Work out the finished part from the listing and answer in its coordinate system (mm). Round coordinates to 2 decimals unless told otherwise and drop trailing zeros. Order: outer loops, then holes, each group sorted by start corner. A loop starts at its lowest first (then second) coordinate and runs counter-clockwise, first axis right, second up. Notation, with made-up numbers: (73.25, -19.5) -> (120.25, -19.5) arc R21 cw to (120.25, -8.5) -> close; hole circle Ø10 at (14.25, 56). An arc over 180 degrees is marked (long way). Use one line per item in the form item = value.
```python
from build123d import *

# Parameters (mm, degrees)
F0_R     = 3.25
F0_R_2   = 0.335
F1_DEPTH = 57.25
F2_SIZE  = 2
F3_SIZE  = 1


with BuildPart() as f1:
    # F0 (on Top) → F1 (new body)
    with BuildSketch(Plane.XY):
        Circle(F0_R)
        Circle(F0_R_2, mode=Mode.SUBTRACT)
    extrude(amount=F1_DEPTH)

    # F2
    f2_edges = [f1.edges().sort_by_distance(p)[0] for p in [
        (-0.335, 0, 57.25),
    ]]
    chamfer(f2_edges, length=F2_SIZE)

    # F3
    f3_edges = [f1.edges().sort_by_distance(p)[0] for p in [
        (-3.25, 0, 0),
    ]]
    chamfer(f3_edges, length=F3_SIZE)


solid = f1.part
```
Item 1: The part is cut by section A-A, the plane z = 42.5. Give the vertices of the cut face in (x, y) (3 decimals), and give its area (3 significant figures).
Findings:
outline = circle Ø6.5 at (0, 0); hole circle Ø0.67 at (0, 0)
area = 32.8 mm^2
Item 2: Consider line 1 along Y through (x, z) = (0, 21) (3 decimals); line 2 along X through (y, z) = (2.25, 12.5); line 3 along X through (y, z) = (-2, 38.5). Determine where each line is inside the solid, lowest interval first.
Findings:
line_1 = -3.25 to -0.335, 0.335 to 3.25
line_2 = -2.35 to 2.35
line_3 = -2.56 to 2.56
Item 3: Flat-ended cylindrical pins translate along their axes: P1, Ø3, axis at x = 2.5, z = 16, coming from the +Y side; P2, Ø3, axis at y = -2, z = 48, coming from the +X side. Find the tip coordinate at first contact, or state that the pin passes through.
Findings:
P1 = 3.09
P2 = 3.21
